from build123d import *

# Parameters (mm, degrees)
SKETCH_1_W          = 223.9
SKETCH_1_H          = 400
EXTRUDE_1_DEPTH     = 4.5
SKETCH_2_R          = 2
SKETCH_2_W          = 8.5
SKETCH_2_H          = 41
CUT_EXTRUDE_1_DEPTH = 10
CUT_EXTRUDE_2_REACH = 460.423
SKETCH_3_R          = 1.6


with BuildPart() as part:
    # 草图1 → 凸台-拉伸1 (new body)
    with BuildSketch(Plane(origin=(0, 0, 0), x_dir=(0, 0, -1), z_dir=(1, 0, 0))):
        with Locations((-111.95, 200)):
            Rectangle(SKETCH_1_W, SKETCH_1_H)
    extrude(amount=EXTRUDE_1_DEPTH)

    # 草图2 → 切除-拉伸1 (cut)
    with BuildSketch(Plane(origin=(4.5, 0, 0), x_dir=(0, 0, -1), z_dir=(1, 0, 0))):
        with Locations((-204.4, 310)):
            Circle(SKETCH_2_R)
        with Locations((-204.4, 286)):
            Circle(SKETCH_2_R)
        with Locations((-204.4, 54)):
            Circle(SKETCH_2_R)
        with Locations((-204.4, 30)):
            Circle(SKETCH_2_R)
        with Locations((-54, 384)):
            Circle(SKETCH_2_R)
        with Locations((-30, 384)):
            Circle(SKETCH_2_R)
        with Locations((-23, 320)):
            Circle(SKETCH_2_R)
        with Locations((-23, 300)):
            Circle(SKETCH_2_R)
        with Locations((-23, 50)):
            Circle(SKETCH_2_R)
        with Locations((-23, 30)):
            Circle(SKETCH_2_R)
        with Locations((-4.25, 310)):
            Rectangle(SKETCH_2_W, SKETCH_2_H)
        with Locations((-4.25, 40)):
            Rectangle(SKETCH_2_W, SKETCH_2_H)
    extrude(amount=-CUT_EXTRUDE_1_DEPTH, mode=Mode.SUBTRACT)

    # 草图3 → 切除-拉伸2 (cut, up to next)
    with BuildSketch(Plane(origin=(4.5, 0, 0), x_dir=(0, 0, -1), z_dir=(1, 0, 0)), mode=Mode.PRIVATE) as cut_extrude_2_sk1:
        with Locations((-211.5, 175)):
            Circle(SKETCH_3_R)
    cut_extrude_2_tool1 = extrude(cut_extrude_2_sk1.sketch, amount=-CUT_EXTRUDE_2_REACH, mode=Mode.PRIVATE) & part.part
    # 草图3 → 切除-拉伸2 (cut, up to next)
    with BuildSketch(Plane(origin=(4.5, 0, 0), x_dir=(0, 0, -1), z_dir=(1, 0, 0)), mode=Mode.PRIVATE) as cut_extrude_2_sk2:
        with Locations((-211.5, 235)):
            Circle(SKETCH_3_R)
    cut_extrude_2_tool2 = extrude(cut_extrude_2_sk2.sketch, amount=-CUT_EXTRUDE_2_REACH, mode=Mode.PRIVATE) & part.part
    # 草图3 → 切除-拉伸2 (cut, up to next)
    with BuildSketch(Plane(origin=(4.5, 0, 0), x_dir=(0, 0, -1), z_dir=(1, 0, 0)), mode=Mode.PRIVATE) as cut_extrude_2_sk3:
        with Locations((-211.5, 115)):
            Circle(SKETCH_3_R)
    cut_extrude_2_tool3 = extrude(cut_extrude_2_sk3.sketch, amount=-CUT_EXTRUDE_2_REACH, mode=Mode.PRIVATE) & part.part
    # 草图3 → 切除-拉伸2 (cut, up to next)
    with BuildSketch(Plane(origin=(4.5, 0, 0), x_dir=(0, 0, -1), z_dir=(1, 0, 0)), mode=Mode.PRIVATE) as cut_extrude_2_sk4:
        with Locations((-173.9, 297.6)):
            Circle(SKETCH_3_R)
    cut_extrude_2_tool4 = extrude(cut_extrude_2_sk4.sketch, amount=-CUT_EXTRUDE_2_REACH, mode=Mode.PRIVATE) & part.part
    # 草图3 → 切除-拉伸2 (cut, up to next)
    with BuildSketch(Plane(origin=(4.5, 0, 0), x_dir=(0, 0, -1), z_dir=(1, 0, 0)), mode=Mode.PRIVATE) as cut_extrude_2_sk5:
        with Locations((-53.9, 297.6)):
            Circle(SKETCH_3_R)
    cut_extrude_2_tool5 = extrude(cut_extrude_2_sk5.sketch, amount=-CUT_EXTRUDE_2_REACH, mode=Mode.PRIVATE) & part.part
    # 草图3 → 切除-拉伸2 (cut, up to next)
    with BuildSketch(Plane(origin=(4.5, 0, 0), x_dir=(0, 0, -1), z_dir=(1, 0, 0)), mode=Mode.PRIVATE) as cut_extrude_2_sk6:
        with Locations((-53.9, 52.4)):
            Circle(SKETCH_3_R)
    cut_extrude_2_tool6 = extrude(cut_extrude_2_sk6.sketch, amount=-CUT_EXTRUDE_2_REACH, mode=Mode.PRIVATE) & part.part
    # 草图3 → 切除-拉伸2 (cut, up to next)
    with BuildSketch(Plane(origin=(4.5, 0, 0), x_dir=(0, 0, -1), z_dir=(1, 0, 0)), mode=Mode.PRIVATE) as cut_extrude_2_sk7:
        with Locations((-173.9, 52.4)):
            Circle(SKETCH_3_R)
    cut_extrude_2_tool7 = extrude(cut_extrude_2_sk7.sketch, amount=-CUT_EXTRUDE_2_REACH, mode=Mode.PRIVATE) & part.part
    # 草图3 → 切除-拉伸2 (cut, up to next)
    with BuildSketch(Plane(origin=(4.5, 0, 0), x_dir=(0, 0, -1), z_dir=(1, 0, 0)), mode=Mode.PRIVATE) as cut_extrude_2_sk8:
        with Locations((-113.9, 297.6)):
            Circle(SKETCH_3_R)
    cut_extrude_2_tool8 = extrude(cut_extrude_2_sk8.sketch, amount=-CUT_EXTRUDE_2_REACH, mode=Mode.PRIVATE) & part.part
    # 草图3 → 切除-拉伸2 (cut, up to next)
    with BuildSketch(Plane(origin=(4.5, 0, 0), x_dir=(0, 0, -1), z_dir=(1, 0, 0)), mode=Mode.PRIVATE) as cut_extrude_2_sk9:
        with Locations((-113.9, 52.4)):
            Circle(SKETCH_3_R)
    cut_extrude_2_tool9 = extrude(cut_extrude_2_sk9.sketch, amount=-CUT_EXTRUDE_2_REACH, mode=Mode.PRIVATE) & part.part
    # 草图3 → 切除-拉伸2 (cut, up to next)
    with BuildSketch(Plane(origin=(4.5, 0, 0), x_dir=(0, 0, -1), z_dir=(1, 0, 0)), mode=Mode.PRIVATE) as cut_extrude_2_sk10:
        with BuildLine():
            Line((-64.4, 74), (-163.4, 74))
            ThreePointArc((-163.4, 74), (-183.198989873, 82.201010127), (-191.4, 102))
            Line((-191.4, 102), (-191.4, 248))
            ThreePointArc((-191.4, 248), (-183.198989873, 267.798989873), (-163.4, 276))
            Line((-163.4, 276), (-64.4, 276))
            ThreePointArc((-64.4, 276), (-44.601010127, 267.798989873), (-36.4, 248))
            Line((-36.4, 248), (-36.4, 102))
            ThreePointArc((-36.4, 102), (-44.601010127, 82.201010127), (-64.4, 74))
        make_face()
    cut_extrude_2_tool10 = extrude(cut_extrude_2_sk10.sketch, amount=-CUT_EXTRUDE_2_REACH, mode=Mode.PRIVATE) & part.part
    add(cut_extrude_2_tool1.solids().sort_by_distance((4.5, 175, 211.5))[0], mode=Mode.SUBTRACT)
    add(cut_extrude_2_tool2.solids().sort_by_distance((4.5, 235, 211.5))[0], mode=Mode.SUBTRACT)
    add(cut_extrude_2_tool3.solids().sort_by_distance((4.5, 115, 211.5))[0], mode=Mode.SUBTRACT)
    add(cut_extrude_2_tool4.solids().sort_by_distance((4.5, 297.6, 173.9))[0], mode=Mode.SUBTRACT)
    add(cut_extrude_2_tool5.solids().sort_by_distance((4.5, 297.6, 53.9))[0], mode=Mode.SUBTRACT)
    add(cut_extrude_2_tool6.solids().sort_by_distance((4.5, 52.4, 53.9))[0], mode=Mode.SUBTRACT)
    add(cut_extrude_2_tool7.solids().sort_by_distance((4.5, 52.4, 173.9))[0], mode=Mode.SUBTRACT)
    add(cut_extrude_2_tool8.solids().sort_by_distance((4.5, 297.6, 113.9))[0], mode=Mode.SUBTRACT)
    add(cut_extrude_2_tool9.solids().sort_by_distance((4.5, 52.4, 113.9))[0], mode=Mode.SUBTRACT)
    add(cut_extrude_2_tool10.solids().sort_by_distance((4.5, 175, 113.9))[0], mode=Mode.SUBTRACT)


solid = part.part
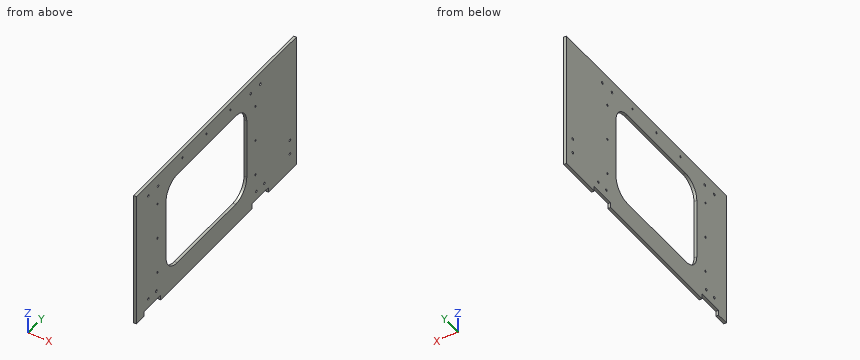
Design review of the part built by this model. Coordinates are the model's own, in mm. Round coordinates to 2 decimals unless told otherwise and drop trailing zeros. Write each loop counter-clockwise with the first axis right and the second up, starting at its lowest first coordinate (ties: lowest second). Pieces come first, ordered by that corner, then holes. Notation, with made-up numbers: (31, 1) - (87, 1) arc R23 cw to (87, 36) - close; hole circle Ø4 at (42, 76). An arc over 180 degrees is marked (long way). Return JSON: item names as keys, results as strings. Group by question number.
Item 1: We need section B-B on y = 106.5. Write out the cut boundary in (x, z).
Item 2: We need section A-A on z = 136. Write out the cut boundary in (x, y), and give its area (3 significant figures).
Item 3: For probe 1 along Y at (x, z) = (1.7, 204.4); probe 2 along Y at (x, z) = (1.3, 113.9); probe 3 along Y at (x, z) = (3.25, 23), list the stretches that pass through material, from the lowest coordinate up. Write a range as [from, to].
Item 4: Insertion check: P1, Ø2, axis at x = 1.5, y = 34.5, coming from the -Z side; P2, Ø3, axis at y = 30, z = 204.4, coming from the -X side; P3, Ø1.3, axis at x = 1.5, z = 5, coming from the -Y side. Each pin has a flat end and moves straight along its axis. Give the tip position at first contact, or say it passes through.
Item 5: We need section C-C on x = 1.8. Give the number of separate pieces and of enclosed holes in the cut face, and give its area (3 significant figures).
Model answer:
{
 "1": {"outline": "(0, 0) - (4.5, 0) - (4.5, 36.4) - (0, 36.4) - close; (0, 191.4) - (4.5, 191.4) - (4.5, 223.9) - (0, 223.9) - close"},
 "2": {"outline": "(0, 0) - (4.5, 0) - (4.5, 74) - (0, 74) - close; (0, 276) - (4.5, 276) - (4.5, 400) - (0, 400) - close", "area": "891 mm²"},
 "3": {"probe 1": "y = [0, 28], [32, 52], [56, 284], [288, 308], [312, 400]", "probe 2": "y = [0, 50.8], [54, 74], [276, 296], [299.2, 400]", "probe 3": "y = [0, 28], [32, 48], [52, 298], [302, 318], [322, 400]"},
 "4": {"P1": "stops at z = 8.5", "P2": "passes through", "P3": "stops at y = 0"},
 "5": {"separate pieces": "1", "enclosed holes": "20", "area": "58,000 mm²"}
}
